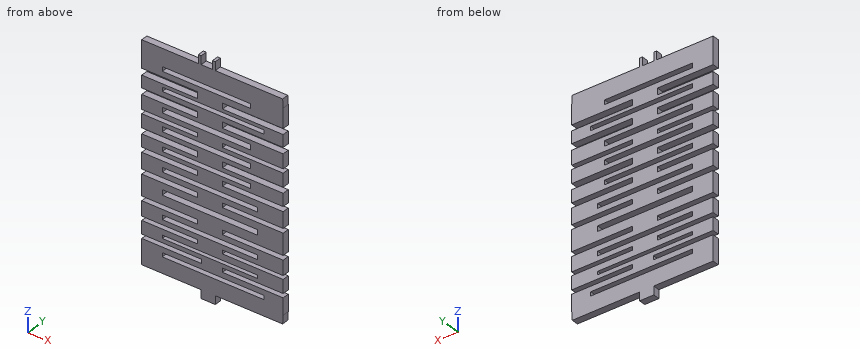
from build123d import *

# Parameters (mm, degrees)
F0_W     = 42.64751
F0_H     = 1.470603
F0_H_2   = 2.02208
F0_H_3   = 2.389731
F0_W_2   = 45.754235
F0_H_4   = 1.838255
F0_W_3   = 39.522478
F0_H_5   = 2.245025
F0_H_6   = 2.022082
F0_H_7   = 1.838256
F1_DEPTH = 3


with BuildPart() as f1:
    # F0 (on Front) → F1 (new body)
    with BuildSketch(Plane.XZ):
        Polygon((-54.974343, 33.532223), (-54.974343, 29.722223), (8.525657, 29.722223), (8.290456, 33.532223), (-21.954343, 33.532223), (-21.954343, 37.342223), (-23.224343, 37.342223), (-23.224343, 33.532223), (-28.304343, 33.532223), (-28.304343, 37.342223), (-29.574343, 37.342223), (-29.574343, 33.532223), align=None)
        Polygon((8.525657, 29.722223), (-54.974343, 29.722223), (-54.974343, 21.275444), (-29.945243, 21.275444), (-29.945243, 18.343428), (-54.974343, 18.343428), (-54.974343, 12.828665), (-29.945243, 12.828665), (-29.945243, 10.071282), (-54.974343, 10.071282), (-54.974343, 3.63739), (-29.945243, 3.63739), (-29.945243, 1.799135), (-54.974343, 1.799135), (-54.974343, -4.267105), (-29.945243, -4.267105), (-29.945243, -6.840662), (-54.974343, -6.840662), (-54.974343, -12.539252), (-29.945243, -12.539252), (-29.945243, -14.727777), (-54.974343, -14.727777), (-54.974343, -21.91435), (-29.945243, -21.91435), (-29.945243, -24.120256), (-54.974343, -24.120256), (-54.974343, -33.495355), (-29.945243, -33.495355), (-29.945243, -35.517436), (-54.974343, -35.517436), (-54.974343, -42.135153), (-29.945243, -42.135153), (-29.945243, -43.973409), (-54.974343, -43.973409), (-54.974343, -49.855825), (-28.106989, -49.855825), (-28.106989, -51.694077), (-54.974343, -51.694077), (-54.974343, -59.177777), (8.525657, -59.177777), (8.525657, -51.694077), (-18.73189, -51.694077), (-18.73189, -49.855825), (8.525657, -49.855825), (8.525657, -43.789584), (-18.73189, -43.789584), (-18.73189, -42.135153), (8.525657, -42.135153), (8.525657, -35.517436), (-18.73189, -35.517436), (-18.73189, -33.495355), (8.525657, -33.495355), (8.525657, -23.936432), (-18.73189, -23.936432), (-18.73189, -21.91435), (8.525657, -21.91435), (8.525657, -14.727777), (-18.73189, -14.727777), (-18.73189, -12.539252), (8.525657, -12.539252), (8.525657, -6.840662), (-18.73189, -6.840662), (-18.73189, -4.267105), (8.525657, -4.267105), (8.525657, 1.799135), (-18.73189, 1.799135), (-18.73189, 3.63739), (8.525657, 3.63739), (8.525657, 10.071282), (-18.73189, 10.071282), (-18.73189, 12.828665), (8.525657, 12.828665), (8.525657, 18.343428), (-18.73189, 18.343428), (-18.73189, 20.916985), (8.525657, 20.916985), align=None)
        with Locations((-24.43048, -47.282267)):
            Rectangle(F0_W, F0_H, mode=Mode.SUBTRACT)
        with Locations((-24.43048, -38.918208)):
            Rectangle(F0_W, F0_H_2, mode=Mode.SUBTRACT)
        with Locations((-24.43048, -28.256329)):
            Rectangle(F0_W, F0_H_3, mode=Mode.SUBTRACT)
        with Locations((-24.43048, -18.513579)):
            Rectangle(F0_W, F0_H_2, mode=Mode.SUBTRACT)
        with Locations((-22.877118, -55.002933)):
            Rectangle(F0_W_2, F0_H_4, mode=Mode.SUBTRACT)
        with Locations((-25.992996, -9.689957)):
            Rectangle(F0_W_3, F0_H_2, mode=Mode.SUBTRACT)
        with Locations((-25.992996, -1.122513)):
            Rectangle(F0_W_3, F0_H_5, mode=Mode.SUBTRACT)
        with Locations((-25.992996, 7.038161)):
            Rectangle(F0_W_3, F0_H_3, mode=Mode.SUBTRACT)
        with Locations((-25.992996, 24.685406)):
            Rectangle(F0_W_3, F0_H_6, mode=Mode.SUBTRACT)
        with Locations((-22.877118, 15.953697)):
            Rectangle(F0_W_2, F0_H_7, mode=Mode.SUBTRACT)
        Polygon((8.525657, -59.177777), (-54.974343, -59.177777), (-54.974343, -62.987777), (-28.304343, -62.987777), (-28.304343, -66.797777), (-21.954343, -66.797777), (-21.954343, -62.987777), (8.290456, -62.987777), align=None)
    extrude(amount=F1_DEPTH)


solid = f1.part
Read the model definition and answer for the solid it produces. Units are mm, in the model's axes. Coordinates: 2 decimals unless noted, no trailing zeros. Answer in a Markdown table with one row per item.
Q1. Given P1, Ø1.5, axis at x = -15, y = -1.5, coming from the -Z side; P2, Ø1.5, axis at y = -1, z = -51, coming from the +X side; P3, Ø0.9, axis at y = -1.5, z = -43, coming from the -X side; P4, Ø1.5, axis at y = -1.5, z = 35, coming from the +X side, each flat-ended and moving along its own axis, determine where each tip first touches the part or whether it passes through.
Here are the results:
| item | result |
|---|---|
| P1 | stops at z = -62.99 |
| P2 | stops at x = 8.53 |
| P3 | stops at x = -29.95 |
| P4 | stops at x = -21.95 |
Q2. Find section A-A on x = -47. Count the separate pieces of the cut face and the enclosed holes in it, plus the area to 3 significant figures.
Here are the results:
| item | result |
|---|---|
| separate pieces | 10 |
| enclosed holes | 0 |
| area | 229 mm^2 |
Q3. Straight lines are drawn through the part: line 1 along X through (y, z) = (-0.4, 25.5); line 2 along X through (y, z) = (-1.4, 3); line 3 along X through (y, z) = (-0.25, 31). For each, find the intervals that lie inside material, in ascending order. Write a range as [from, to].
Here are the results:
| item | result |
|---|---|
| line 1 | x = [-54.97, -45.75], [-6.23, 8.53] |
| line 2 | x = [-29.95, -18.73] |
| line 3 | x = [-54.97, 8.45] |
